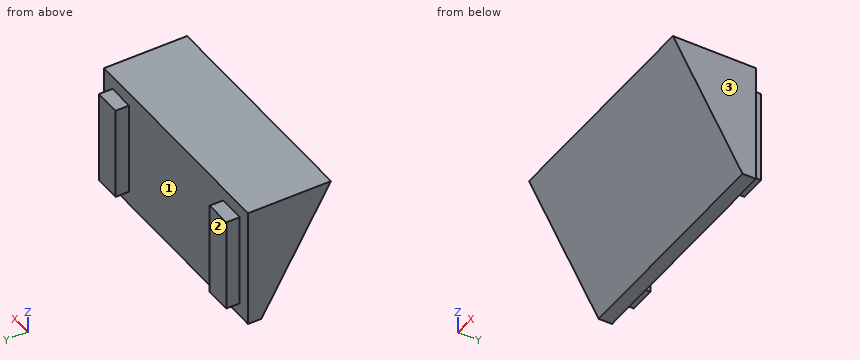
from build123d import *

# Parameters (mm, degrees)
SKETCH1_W             = 6
SKETCH1_H             = 21
BOSS_EXTRUDE1_DEPTH   = 3
BOSS_EXTRUDE1_2_DEPTH = 3
SKETCH1_3_W           = 52
SKETCH1_3_H           = 27
SKETCH1_3_W_2         = 46
SKETCH1_3_H_2         = 21
SKETCH1_3_W_3         = 34
SKETCH1_3_W_4         = 6
BOSS_EXTRUDE2_DEPTH   = 3
BOSS_EXTRUDE3_DEPTH   = 52


with BuildPart() as part:
    # Sketch1 → Boss-Extrude1 (new body)
    with BuildSketch(Plane(origin=(0, 0, 0), x_dir=(1, 0, 0), z_dir=(0, 1, 0))):
        with Locations((-20, 0)):
            Rectangle(SKETCH1_W, SKETCH1_H)
    extrude(amount=BOSS_EXTRUDE1_DEPTH)



with BuildPart() as body_2:
    # Sketch1 → Boss-Extrude1 2 (new body)
    with BuildSketch(Plane(origin=(0, 0, 0), x_dir=(1, 0, 0), z_dir=(0, 1, 0))):
        with Locations((20, 0)):
            Rectangle(SKETCH1_W, SKETCH1_H)
    extrude(amount=BOSS_EXTRUDE1_2_DEPTH)


with BuildPart() as body_3:
    # Sketch1_3 → Boss-Extrude2 (new body)
    # profile 1 of 4: a face of its own
    with BuildSketch(Plane(origin=(0, 0, 0), x_dir=(1, 0, 0), z_dir=(0, 1, 0))):
        Rectangle(SKETCH1_3_W, SKETCH1_3_H)
        Rectangle(SKETCH1_3_W_2, SKETCH1_3_H_2, mode=Mode.SUBTRACT)
    # profile 2 of 4: a face of its own
    with BuildSketch(Plane(origin=(0, 0, 0), x_dir=(1, 0, 0), z_dir=(0, 1, 0))):
        Rectangle(SKETCH1_3_W_3, SKETCH1_3_H_2)
    # profile 3 of 4: a face of its own
    with BuildSketch(Plane(origin=(0, 0, 0), x_dir=(1, 0, 0), z_dir=(0, 1, 0))):
        with Locations((-20, 0)):
            Rectangle(SKETCH1_3_W_4, SKETCH1_3_H_2)
    # profile 4 of 4: a face of its own
    with BuildSketch(Plane(origin=(0, 0, 0), x_dir=(1, 0, 0), z_dir=(0, 1, 0))):
        with Locations((20, 0)):
            Rectangle(SKETCH1_3_W_4, SKETCH1_3_H_2)
    extrude(amount=-BOSS_EXTRUDE2_DEPTH)


with BuildPart() as part_1:
    add(part.part)

    add(body_2.part)  # Boss-Extrude3 merges body 2

    add(body_3.part)  # Boss-Extrude3 merges body 3
    # Sketch2 → Boss-Extrude3 (add)
    with BuildSketch(Plane.ZY.offset(26)):
        Polygon((13.5, -3), (13.5, -18.588457268), (-13.5, -3), (-13.5, 0), (13.5, 0), align=None)
    extrude(amount=-BOSS_EXTRUDE3_DEPTH)


solid = part_1.part
CAD build for the part. Positions are in the model's coordinates, mm. Face numbers are marked on the shaded views. Round coordinates to 2 decimals unless told otherwise and drop trailing zeros. Loops run counter-clockwise (first coordinate to the right, second up) from the corner with the lowest first, then second, coordinate; pieces in that order, holes last. Notation, with made-up numbers: (66, -2) - (98, -2) arc R18 cw to (98, 8) - close; hole circle Ø6 at (76.5, 0.25). An arc over 180 degrees is marked (long way). Put each result on its own line as item: value.
1. Two-plate mould, pull along X, no slides. Class the marked faces 1, 2 and 3: released by +X, released by -X, zero draft, split by the parting line, or undercut.
Geometry check:
face 1: undercut
face 2: zero draft
face 3: released by +X
2. Pin check, flat tips, straight feed: P1, Ø1.5, axis at y = 2, z = -3, coming from the +X side; P2, Ø3.5, axis at x = 19, y = 2, coming from the -Z side; P3, Ø1.5, axis at y = 1, z = -4.5, coming from the -X side. Stop position of each tip, or through.
Geometry check:
P1: x = 23
P2: z = -10.5
P3: x = -23
3. Slice it at D-D on z = 0. List the corners of the cut face in (x, y), and give its area (3 significant figures).
Geometry check:
outline: (-26, -10.79) - (26, -10.79) - (26, 0) - (23, 0) - (23, 3) - (17, 3) - (17, 0) - (-17, 0) - (-17, 3) - (-23, 3) - (-23, 0) - (-26, 0) - close
area: 597 mm²
4. Slice it at A-A on x = 22.5. List the corners of the cut face in (y, z), and give its area (3 significant figures).
Geometry check:
outline: (-18.59, 13.5) - (-3, -13.5) - (0, -13.5) - (0, -10.5) - (3, -10.5) - (3, 10.5) - (0, 10.5) - (0, 13.5) - close
area: 354 mm²
5. Wall check: line 1 (X direction, y = 1.5, z = 4.75); line 2 (Z direction, x = 5, y = -17.25); line 3 (Z direction, x = -21.5, y = -11.75). Give the ranges that are in metal, low to high.
Geometry check:
line 1: -23 to -17, 17 to 23
line 2: 11.18 to 13.5
line 3: 1.66 to 13.5
6. Slice it at C-C on y = -16. List the corners of the cut face in (x, z).
Geometry check:
outline: (-26, 9.02) - (26, 9.02) - (26, 13.5) - (-26, 13.5) - close
7. Slice it at B-B on z = -8. List the corners of the cut face in (x, y), and give its area (3 significant figures).
Geometry check:
outline: (-26, -6.18) - (26, -6.18) - (26, 0) - (23, 0) - (23, 3) - (17, 3) - (17, 0) - (-17, 0) - (-17, 3) - (-23, 3) - (-23, 0) - (-26, 0) - close
area: 357 mm²
